Work out the finished part from the listing and answer in its coordinate system (mm). A direction names the side the tool comes from. Give positions to 0.01 mm unless a question says otherwise; leave off trailing zeros. Loops run counter-clockwise (first coordinate to the right, second up) from the corner with the lowest first, then second, coordinate; pieces in that order, holes last. Notation, with made-up numbers: (24.25, 80) - (67.25, 80) arc R22 ccw to (67.25, 116) - close; hole circle Ø9 at (-0.5, -29.75). An arc over 180 degrees is marked (long way). One line per question, with ' | ' between items. Start each with the question number.
1. Section C-C (z = 51.5) is taken. Determine the outline of the cut face in (x, y).
2. Section B-B (y = 0) is taken. Determine the outline of the cut face in (x, z), plus the area to 3 significant figures.
3. Which of the six approach directions +Z, -Z, +X, -X, +Y, -Y give full straight-line access (tool end or side, diameter ignored) to faces 1 (the face through (51, -3, 7.938)), 2 (the face through (57.15, -34, 5)), 3 (the face through (57.15, 38, 22)), 4 (the face through (29, -41, 4)), 5 (the face through (133.345, -0.489, 3.913))?
4. For a pull along X with two mould halves and no side action, classify faces 6 (the face through (28, 36.512, 33)), 7 (the face through (0, -0.6, 7.7)), 8 (the face through (26.424, 40.537, 34.763)), 9 (the face through (29.2, 40.43, 73.02)) as released by +X, released by -X, zero draft, split by the parting line, or undercut.
5. Each of these flat-tipped pins is pushed along its axis until it touches: pin 1 (23.5 mm diameter, centred on x = 111.125, y = 0, fed in from -Z); pin 2 (16 mm diameter, centred on x = 28.575, z = 44.45, fed in from -Y); pin 3 (2.5 mm diameter, centred on x = 88, z = 6, fed in from +Y) (3 decimals); pin 4 (8.5 mm diameter, centred on x = 76.5, z = 5, fed in from -Y) (3 decimals). Where does it stop, or does it pass through?
6. Section A-A (z = 31.5) is taken. Determine the outline of the cut face in (x, y), plus the area to 3 significant figures.
7. Find the intervals of material crossed by line 1 (Y direction, x = 11.5, z = 55); line 2 (X direction, y = 40, z = 44); line 3 (Z direction, x = 109.5, y = -21), in increasing order.
from build123d import *

# Parameters (mm, degrees)
F0_R     = 10.3251
F1_DEPTH = 7.9375
F2_R     = 9.92251
F3_DEPTH = 44.45
F4_W     = 73.025
F4_H     = 78.11679
F5_DEPTH = 133.351001
F6_R     = 12.7


with BuildPart() as f1:
    # F0 (on Top) → F1 (new body)
    with BuildSketch(Plane.XY):
        with BuildLine():
            Line((57.15, 44.45), (0, 44.45))
            Line((0, 44.45), (0, -44.45))
            Line((0, -44.45), (57.150001, -44.45))
            Line((57.150001, -44.45), (57.150001, -28.575))
            ThreePointArc((57.150001, -28.575), (59.009873, -24.084872), (63.5, -22.225))
            Line((63.5, -22.225), (111.125001, -22.225))
            ThreePointArc((111.125001, -22.225), (133.350001, 0), (111.125001, 22.225))
            Line((111.125001, 22.225), (63.5, 22.225))
            ThreePointArc((63.5, 22.225), (59.009872, 24.084872), (57.15, 28.575))
            Line((57.15, 28.575), (57.15, 44.45))
        make_face()
        with Locations((73.025001, 0)):
            Circle(F0_R, mode=Mode.SUBTRACT)
        with Locations((111.125001, 0)):
            Circle(F0_R, mode=Mode.SUBTRACT)
    extrude(amount=F1_DEPTH)

    # F2 (on Front) → F3 (join, symmetric)
    with BuildSketch(Plane.XZ):
        with BuildLine():
            Line((0, 44.45), (0, 7.9375))
            Line((0, 7.9375), (57.15, 7.9375))
            Line((57.15, 7.9375), (57.15, 44.45))
            ThreePointArc((57.15, 44.45), (28.575, 73.025), (0, 44.45))
        make_face()
        with Locations((28.575, 44.45)):
            Circle(F2_R, mode=Mode.SUBTRACT)
    extrude(amount=F3_DEPTH, both=True)

    # F4 (on face) → F5 (cut, through all)
    with BuildSketch(Plane(origin=(0, 0, 0), x_dir=(0, -1, 0), z_dir=(-1, 0, 0))):
        with Locations((0, 46.995895)):
            Rectangle(F4_W, F4_H)
    extrude(amount=-F5_DEPTH, mode=Mode.SUBTRACT)

    # F6
    f6_edges = [f1.edges().sort_by_distance(p)[0] for p in [
        (28.575001, -44.45, 0),
        (28.575, 44.45, 0),
    ]]
    fillet(f6_edges, radius=F6_R)


solid = f1.part
Conclusion:
1) outline: (0.88, -44.45) - (21.59, -44.45) - (21.59, -36.51) - (0.88, -36.51) - close; (0.88, 36.51) - (21.59, 36.51) - (21.59, 44.45) - (0.88, 44.45) - close; (35.56, -44.45) - (56.27, -44.45) - (56.27, -36.51) - (35.56, -36.51) - close; (35.56, 36.51) - (56.27, 36.51) - (56.27, 44.45) - (35.56, 44.45) - close
2) outline: (0, 0) - (62.7, 0) - (62.7, 7.94) - (0, 7.94) - close; (83.35, 0) - (100.8, 0) - (100.8, 7.94) - (83.35, 7.94) - close; (121.45, 0) - (133.35, 0) - (133.35, 7.94) - (121.45, 7.94) - close | area: 731 mm²
3) face 1: +Z, +X, -X | face 2: +Z, -Z, +X, -Y | face 3: +Z, -Z, +X, +Y | face 4: -Z, +X, -X, -Y | face 5: +Z, -Z, +X
4) face 6: zero draft | face 7: released by -X | face 8: undercut | face 9: split by the parting line
5) pin 1: z = 0 | pin 2: through | pin 3: y = 22.225 | pin 4: y = -22.225
6) outline: (0, -44.45) - (57.15, -44.45) - (57.15, -36.51) - (0, -36.51) - close; (0, 36.51) - (57.15, 36.51) - (57.15, 44.45) - (0, 44.45) - close | area: 907 mm²
7) line 1: -44.45 to -36.51, 36.51 to 44.45 | line 2: 0 to 18.66, 38.49 to 57.15 | line 3: 0 to 7.94
